Here's the drawing with two shaded views (mm, measured from the low corner). I have some questions. A direction names the side the tool comes from. Coordinates: 2 decimals unless noted, no trailing zeros. Write each loop counter-clockwise with the first axis right and the second up, starting at its lowest first coordinate (ties: lowest second). Pieces come first, ordered by that corner, then holes. Notation, with made-up numbers: (45, 42) -> (54, 42) arc R27 ccw to (54, 76) -> close; hole circle Ø8 at (80.25, 74.5). An arc over 180 degrees is marked (long way). Answer in a Markdown table with one row per item. Add a question column.
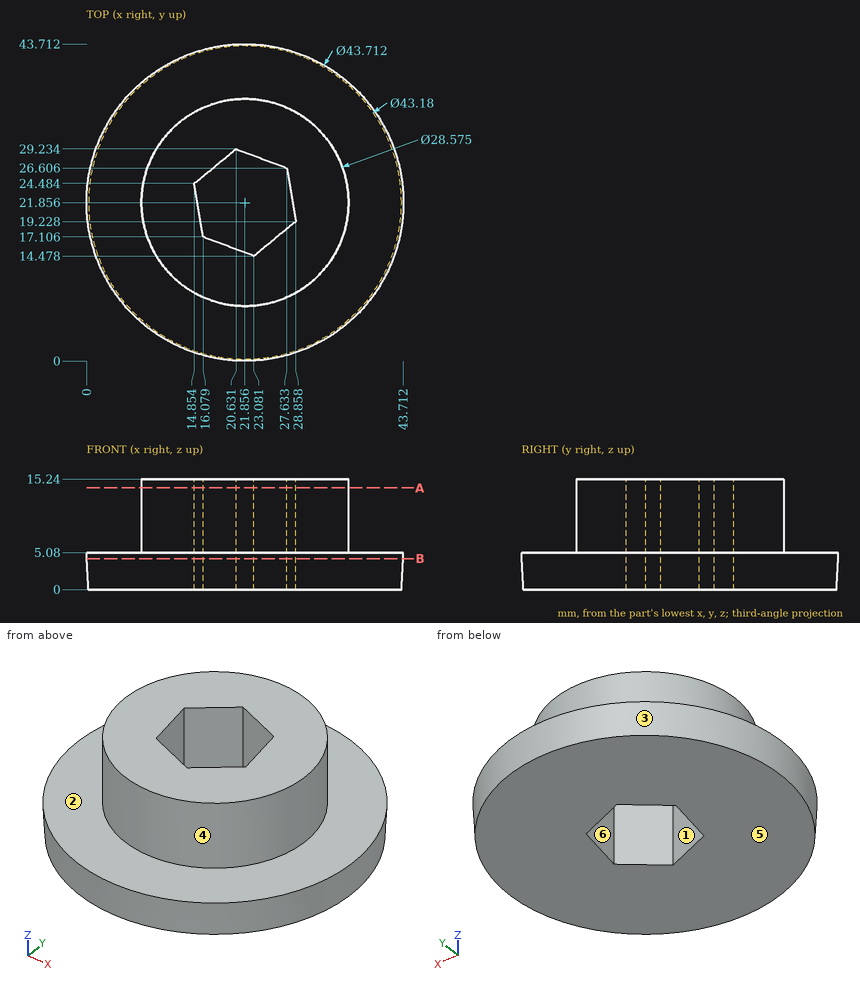
Q1. If we mould it in two halves opening along Y, with no side actions, what happens to the marked faces 4, 5 and 6? For each: pulls with the +Y half, pulls with the -Y half, needs draft (parallel to the pull), parting line crosses it, or undercut.
Q2. I'm going to push flat-ended pins straight in: P1, Ø5, axis at x = 35.5, z = 9, coming from the -Y side (1 decimal); P2, Ø3, axis at x = 36.5, z = 2.5, coming from the -Y side; P3, Ø5, axis at x = 30.5, y = 6, coming from the +Z side. Where does each tip first touch, or does it pass through?
Q3. For the marked faces 1, 2 and 3, which set-ups out of +Z, -Z, +X, -X, +Y, -Y let a thin tool reach every point of the face, with its end or its side?
Q4. Imagine slicing it at A-A on z = 14. Please give me the cut outline in (x, y) (1 decimal), plus the area to 3 significant figures.
Q5. I need wall thicknesses on line 1 (Y direction, x = 26, z = 3.5); line 2 (Y direction, x = 20, z = 10.25) (1 decimal); line 3 (Z direction, x = 17.5, y = 39). Which ranges of each line are inside material? Lowest first, please. Write a range as [from, to].
Q6. Imagine slicing it at B-B on z = 4.25. Please give me the cut outline in (x, y) (1 decimal).
Result sheet:
| question | item | result |
|---|---|---|
| 1 | face 4 | parting line crosses it |
| 1 | face 5 | needs draft |
| 1 | face 6 | undercut |
| 2 | P1 | stops at y = 12.9 |
| 2 | P2 | stops at y = 4.56 |
| 2 | P3 | stops at z = 5.08 |
| 3 | face 1 | +Z, -Z |
| 3 | face 2 | +Z |
| 3 | face 3 | -Z |
| 4 | outline | circle Ø28.6 at (21.9, 21.9); hole (14.9, 24.5) -> (16.1, 17.1) -> (23.1, 14.5) -> (28.9, 19.2) -> (27.6, 26.6) -> (20.6, 29.2) -> close |
| 4 | area | 496 mm^2 |
| 5 | line 1 | y = [0.48, 16.88], [27.22, 43.23] |
| 5 | line 2 | y = [7.7, 15.6], [28.7, 36] |
| 5 | line 3 | z = [0, 5.08] |
| 6 | outline | circle Ø43.6 at (21.9, 21.9); hole (14.9, 24.5) -> (16.1, 17.1) -> (23.1, 14.5) -> (28.9, 19.2) -> (27.6, 26.6) -> (20.6, 29.2) -> close |
